Geometry check sheet. Reference: the model listing, model coordinates, mm. Face numbers are marked on the shaded views. A direction names the side the tool comes from. Round coordinates to 2 decimals unless told otherwise and drop trailing zeros. Write each loop counter-clockwise with the first axis right and the second up, starting at its lowest first coordinate (ties: lowest second). Pieces come first, ordered by that corner, then holes. Notation, with made-up numbers: (4, -38) -> (28, -38) arc R20 cw to (28, -21) -> close; hole circle Ø1 at (87.25, 51). An arc over 180 degrees is marked (long way). Use a Markdown table: item, result.
Autodesk Inventor part; units mm, degrees
ref_plane "YZ Plane" through (0, 0, 0) normal (1, 0, 0) x (0, 1, 0)
ref_plane "XZ Plane" through (0, 0, 0) normal (0, 1, 0) x (-1, 0, 0)
ref_plane "XY Plane" through (0, 0, 0) normal (0, 0, 1) x (1, 0, 0)
sketch "Szkic1" plane through (0, 0, 0) normal (0, 0, 1) x (1, 0, 0)
  line L0 (0, 0) -> (15, 0)
  line L1 (15, 0) -> (15, 11.5)
  line L2 (15, 11.5) -> (0, 11.5)
  line L3 (0, 11.5) -> (0, 0)
  line L4 (1.5, 1.5) -> (13.5, 1.5)
  line L5 (13.5, 1.5) -> (13.5, 10)
  line L6 (13.5, 10) -> (1.5, 10)
  line L7 (1.5, 10) -> (1.5, 1.5)
  line L8 (1.5, 1.5) -> (1.5, 0)
  line L9 (13.5, 1.5) -> (13.5, 0)
  line L10 (0, 0) -> (15, 0)
  line L11 (15, 0) -> (15, -1)
  line L12 (15, -1) -> (0, -1)
  line L13 (0, -1) -> (0, 0)
  line L14 (13.5, 0) -> (13.5, -1)
  line L15 (1.5, 0) -> (1.5, -1)
  dimension "d0" = 15
  dimension "d1" = 11.5
  dimension "d2" = 1.5
  dimension "d3" = 1
extrude "Wyciągnięcie proste1" add sketch "Szkic1" along normal blind 20 contours L3 L2 L1 L0 L9 L5 L6 L7 L8 | L0 L15 L12 L13 | L0 L11 L12 L14
fillet "Zaokrąglenie1" radius 2 2 edges at (15, 11.5, 10) (0, 11.5, 10)
sketch "Szkic2" plane through (13.5, -1, 0) normal (0, -1, 0) x (1, 0, 0)
  line L0 (-13.5, 0) -> (-13.5, 20)
  line L1 (1.5, 0) -> (1.5, 20)
  line L2 (0, 0) -> (1.5, 0)
  circle A0 centre (3, 13) radius 1.25
  circle A1 centre (-15, 13) radius 1.25
  circle A2 centre (3, 13) radius 4.25
  circle A3 centre (-15, 13) radius 4.25
  line L3 (3, 8.75) -> (1.5, 8.75)
  line L4 (-15, 8.75) -> (-13.5, 8.75)
  line L5 (3, 17.25) -> (1.5, 17.25)
  line L6 (-15, 17.25) -> (-13.5, 17.25)
  dimension "d7" = 1.5
  dimension "d8" = 1.5
  dimension "d9" = 13
  dimension "d10" = 2.5
  dimension "d11" = 2.5
  dimension "d12" = 8.5
  dimension "d13" = 8.5
extrude "Wyciągnięcie proste2" add sketch "Szkic2" against normal blind 2 contours L4 A3 L0 | A3 L0 | A3 L6 L0 | L1 A2 L3 | L1 A2 | L1 L5 A2 picked at (-15.3893, 9.7942) picked at (6.2145, 12.6848)
sketch "Szkic3" plane through (0, -1, 0) normal (0, -1, 0) x (1, 0, 0)
  line L0 (1.5, 0) -> (1.5, 20)
  line L1 (1.5, 11) -> (0, 11)
  line L2 (0, 11) -> (0, 15)
  line L3 (0, 15) -> (1.5, 15)
  line L4 (1.5, 15) -> (1.5, 11)
  circle A0 centre (-1.5, 13) radius 1.25
  line L5 (0, 0) -> (0, 20)
  line L6 (-1.5, 11.75) -> (0, 11.75)
  line L7 (0, 11.75) -> (0, 14.25)
  line L8 (0, 14.25) -> (-1.5, 14.25)
  line L9 (-1.5, 14.25) -> (-1.5, 11.75)
  line L10 (13.5, 0) -> (13.5, 20)
  line L11 (13.5, 11) -> (15, 11)
  line L12 (15, 11) -> (15, 15)
  line L13 (15, 15) -> (13.5, 15)
  line L14 (13.5, 15) -> (13.5, 11)
  circle A1 centre (16.5, 13) radius 1.25
  line L15 (16.5, 11.75) -> (15, 11.75)
  line L16 (15, 11.75) -> (15, 14.25)
  line L17 (15, 14.25) -> (16.5, 14.25)
  line L18 (16.5, 14.25) -> (16.5, 11.75)
  dimension "d16" = 1.5
  dimension "d17" = 4
  dimension "d18" = 2
  dimension "d19" = 1.5
  dimension "d20" = 4
extrude "Wyciągnięcie proste3" cut sketch "Szkic3" against normal blind 3.5 contours L1 L2 L3 L0 | L6 A0 L8 L2 | L10 L13 L12 L11 | L12 L17 A1 L15 | L18 A1 | A1 L18
sketch "Szkic4" plane through (13.5, 1, 0) normal (0, 1, 0) x (1, 0, 0)
  arc A0 (-15, -11.75) -> (-15, -14.25) centre (-15, -13) ccw
  arc A1 (3, -14.25) -> (3, -11.75) centre (3, -13) ccw
  arc A2 (3, -17.25) -> (3, -8.75) centre (3, -13) ccw
  line L0 (3, -16) -> (0.4019, -14.5)
  line L1 (0.4019, -14.5) -> (0.4019, -11.5)
  line L2 (0.4019, -11.5) -> (3, -10)
  line L3 (3, -10) -> (5.5981, -11.5)
  line L4 (5.5981, -11.5) -> (5.5981, -14.5)
  line L5 (5.5981, -14.5) -> (3, -16)
  line L6 (-15, -16) -> (-17.5981, -14.5)
  line L7 (-17.5981, -14.5) -> (-17.5981, -11.5)
  line L8 (-17.5981, -11.5) -> (-15, -10)
  line L9 (-15, -10) -> (-12.4019, -11.5)
  line L10 (-12.4019, -11.5) -> (-12.4019, -14.5)
  line L11 (-12.4019, -14.5) -> (-15, -16)
  line L12 (1.5, -11.75) -> (3, -11.75)
  arc A3 (3, -14.25) -> (3, -11.75) centre (3, -13) ccw
  line L13 (3, -14.25) -> (1.5, -14.25)
  line L14 (1.5, -15) -> (1.5, -14.25)
  line L15 (1.5, -17.25) -> (1.5, -15)
  line L16 (1.5, -17.25) -> (3, -17.25)
  arc A4 (3, -17.25) -> (3, -8.75) centre (3, -13) ccw
  line L17 (3, -8.75) -> (1.5, -8.75)
  line L18 (1.5, -11) -> (1.5, -8.75)
  line L19 (1.5, -11.75) -> (1.5, -11)
  line L20 (-15, -11.75) -> (-13.5, -11.75)
  line L21 (-13.5, -11) -> (-13.5, -11.75)
  line L22 (-13.5, -8.75) -> (-13.5, -11)
  line L23 (-13.5, -8.75) -> (-15, -8.75)
  arc A5 (-15, -8.75) -> (-15, -17.25) centre (-15, -13) ccw
  line L24 (-15, -17.25) -> (-13.5, -17.25)
  line L25 (-13.5, -15) -> (-13.5, -17.25)
  line L26 (-13.5, -14.25) -> (-13.5, -15)
  line L27 (-13.5, -14.25) -> (-15, -14.25)
  arc A6 (-15, -11.75) -> (-15, -14.25) centre (-15, -13) ccw
  point P0 (-13.5, 0)
  point P1 (-13.5, -10.866)
  point P2 (-13.5, -15.134)
  point P3 (1.5, -15.134)
  point P4 (1.5, -10.866)
  dimension "d23" = 6
extrude "Wyciągnięcie proste4" add sketch "Szkic4" along normal blind 2 contours L9 L8 L7 L6 L11 L25 L24 A5 L23 L22 | L0 L5 L4 L3 L2 L18 L17 A2 L16 L15
sketch "Szkic5" plane through (1.5, 10, 0) normal (0, -1, 0) x (1, 0, 0)
  arc A0 (-3, 14.25) -> (-3, 11.75) centre (-3, 13) ccw
  arc A1 (15, 11.75) -> (15, 14.25) centre (15, 13) ccw
  line L0 (4, 6.5) -> (12, 6.5)
  line L1 (12, 6.5) -> (12, 8)
  line L2 (12, 8) -> (4, 8)
  line L3 (4, 8) -> (4, 6.5)
  line L4 (12, 0) -> (12, 20)
  point P0 (-1.5, 0)
  point P1 (12, 7.25)
  dimension "d26" = 8
  dimension "d27" = 1.5
  dimension "d28" = 5
extrude "Wyciągnięcie proste5" add sketch "Szkic5" along normal blind 2
sketch "Szkic6" plane through (2, 11.5, 0) normal (0, 1, 0) x (1, 0, 0)
  line L0 (-2, 0) -> (0, 0)
  line L1 (13, 0) -> (13, -8.75)
  line L2 (-2, 0) -> (13, 0)
  line L3 (13, 0) -> (13, -4)
  line L4 (13, -4) -> (-2, -4)
  line L5 (-2, -4) -> (-2, 0)
  dimension "d31" = 4
extrude "Wyciągnięcie proste6" cut sketch "Szkic6" against normal through all
properties part number "mocowanie_silnik"
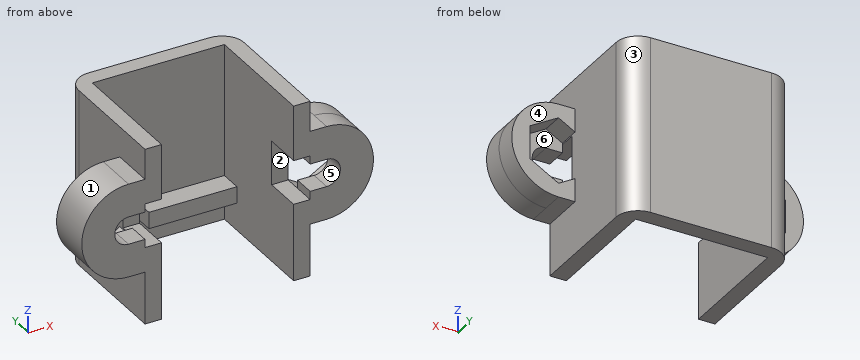
(1) Access from +Z, -Z, +X, -X, +Y, -Y to the whole of each face (thin tool, end or side, straight path). Record for the marked faces 4, 5 and 6.
A:
| item | result |
|---|---|
| face 4 | +Z, -Z, +X, +Y |
| face 5 | +Y, -Y |
| face 6 | +Y |
(2) Release check for a two-part mould opening along Z. For the marked faces 1, 2 and 3 record: +Z half, -Z half, draft (parallel to the pull), parting line (faces both ways), or undercut.
A:
| item | result |
|---|---|
| face 1 | parting line |
| face 2 | undercut |
| face 3 | draft |
(3) Gauge pin test, flat ends, axial feed: pin 1 Ø3 at (x, z) = (10, 12) entering from -Y; pin 2 Ø0.8 at (x, y) = (-0.5, 1) entering from +Z; pin 3 Ø1.2 at (x, z) = (10, 7) entering from -Y. Record the tip position at first contact, or that the pin passes through.
A:
| item | result |
|---|---|
| pin 1 | stops at y = 10 |
| pin 2 | stops at z = 17.25 |
| pin 3 | stops at y = 8 |
(4) Section check B-B on y = 5. Record the cut outline in (x, z), plus the area to 3 significant figures.
A:
| item | result |
|---|---|
| outline | (0, 4) -> (1.5, 4) -> (1.5, 20) -> (0, 20) -> close; (13.5, 4) -> (15, 4) -> (15, 20) -> (13.5, 20) -> close |
| area | 48.0 mm2 |
(5) Section check C-C on x = 12. Record the cut outline in (y, z).
A:
| item | result |
|---|---|
| outline | (8, 6.5) -> (10, 6.5) -> (10, 4) -> (11.5, 4) -> (11.5, 20) -> (10, 20) -> (10, 8) -> (8, 8) -> close |
(6) Thickness scan on line 1 (X direction, y = 4.75, z = 10.25); line 2 (Y direction, x = 16, z = 9.75); line 3 (Y direction, x = 2.5, z = 12.75). Record the ranges inside material, lowest first.
A:
| item | result |
|---|---|
| line 1 | x = 0 to 1.5, 13.5 to 15 |
| line 2 | y = -1 to 3 |
| line 3 | y = 10 to 11.5 |
(7) Section check D-D on z = 5.25. Record the cut outline in (x, y), plus the area to 3 significant figures.
A:
| item | result |
|---|---|
| outline | (0, -1) -> (1.5, -1) -> (1.5, 10) -> (13.5, 10) -> (13.5, -1) -> (15, -1) -> (15, 9.5) arc R2 ccw to (13, 11.5) -> (2, 11.5) arc R2 ccw to (0, 9.5) -> close |
| area | 53.8 mm2 |
(8) Section check A-A on z = 13. Record the cut outline in (x, y), plus the area to 3 significant figures.
A:
| item | result |
|---|---|
| outline | (-5.75, -1) -> (-2.75, -1) -> (-2.75, 1) -> (-4.1, 1) -> (-4.1, 3) -> (-5.75, 3) -> close; (0, 2.5) -> (1.5, 2.5) -> (1.5, 10) -> (13.5, 10) -> (13.5, 2.5) -> (15, 2.5) -> (15, 9.5) arc R2 ccw to (13, 11.5) -> (2, 11.5) arc R2 ccw to (0, 9.5) -> close; (17.75, -1) -> (20.75, -1) -> (20.75, 3) -> (19.1, 3) -> (19.1, 1) -> (17.75, 1) -> close |
| area | 61.9 mm2 |
